Source: three-view drawing plus pictorial views. Frame: mm from the lowest corner of the part. A direction names the side the tool comes from. Give positions to 0.01 mm unless a question says otherwise; leave off trailing zeros. Write each loop counter-clockwise with the first axis right and the second up, starting at its lowest first coordinate (ties: lowest second). Pieces come first, ordered by that corner, then holes. Notation, with made-up numbers: M 54.25,-13.75 L 96.25,-13.75 A28 ccw 96.25,5.25 Z; hole C 44,-2.75 d11. An arc over 180 degrees is marked long. One line per question, with ' | ' between items.
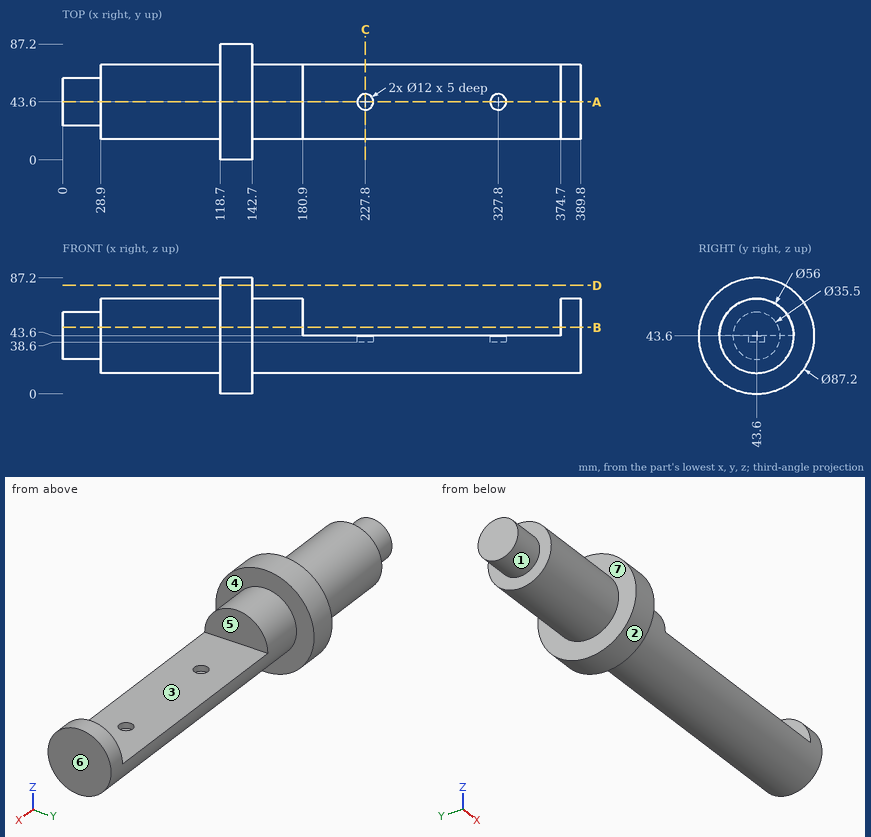
(1) Cut plane B-B, the plane z = 50. Return loops of the section in (x, y).
Working result:
outline: M 0,27.04 L 28.9,27.04 L 28.9,16.34 L 118.7,16.34 L 118.7,0.47 L 142.7,0.47 L 142.7,16.34 L 180.9,16.34 L 180.9,70.86 L 142.7,70.86 L 142.7,86.73 L 118.7,86.73 L 118.7,70.86 L 28.9,70.86 L 28.9,60.16 L 0,60.16 Z; M 374.7,16.34 L 389.8,16.34 L 389.8,70.86 L 374.7,70.86 Z
(2) First-contact query: P1, Ø12, axis at x = 154.5, z = 37, coming from the -Y side; P2, Ø14, axis at x = 327.8, y = 43.6, coming from the -Z side; P3, Ø9.5, axis at x = 229, y = 45, coming from the +Z side. Flat tips, straight axial feed; report the tip coordinate or a pass-through.
Working result:
P1: stops at y = 15.61 | P2: stops at z = 15.6 | P3: stops at z = 43.6
(3) Cut plane C-C, the plane x = 227.8. Return loops of the section in (y, z), then the cut area to 3 significant figures.
Working result:
outline: M 15.6,43.6 A28 ccw 71.6,43.6 L 49.6,43.6 L 49.6,38.6 L 37.6,38.6 L 37.6,43.6 Z | area: 1,170 mm^2
(4) Cut plane A-A, the plane y = 43.6. Return loops of the section in (x, z).
Working result:
outline: M 0,25.85 L 28.9,25.85 L 28.9,15.6 L 118.7,15.6 L 118.7,0 L 142.7,0 L 142.7,15.6 L 389.8,15.6 L 389.8,71.6 L 374.7,71.6 L 374.7,43.6 L 333.8,43.6 L 333.8,38.6 L 321.8,38.6 L 321.8,43.6 L 233.8,43.6 L 233.8,38.6 L 221.8,38.6 L 221.8,43.6 L 180.9,43.6 L 180.9,71.6 L 142.7,71.6 L 142.7,87.2 L 118.7,87.2 L 118.7,71.6 L 28.9,71.6 L 28.9,61.35 L 0,61.35 Z
(5) Material intervals for L1, parallel to X at y = 43, z = 41; L2, parallel to Y at x = 327, z = 42; L3, parallel to X at y = 63, z = 61.5, sorted ascending. Write a range as [from, to].
Working result:
L1: x = [0, 221.83], [233.77, 321.83], [333.77, 389.8] | L2: y = [15.65, 37.65], [49.55, 71.55] | L3: x = [28.9, 180.9], [374.7, 389.8]
(6) Cut plane D-D, the plane z = 81.5. Return loops of the section in (x, y).
Working result:
outline: M 118.7,22.05 L 142.7,22.05 L 142.7,65.15 L 118.7,65.15 Z
(7) Set-up query: the marked faces 1, 2, 3 and 4. Return all of +Z, -Z, +X, -X, +Y, -Y with unobstructed straight access to the full face (end or side cutting, diameter ignored); none if empty.
Working result:
face 1: -X | face 2: +X, -X | face 3: +Z, +Y, -Y | face 4: +X
(8) Draft query along X for the marked faces 5, 6 and 7. Return one class per face: released by +X, released by -X, zero draft, split by the parting line, or undercut.
Working result:
face 5: undercut | face 6: released by +X | face 7: released by -X
